Build history of the part. All positions in model axes, mm. A direction names the side the tool comes from. Round coordinates to 2 decimals unless told otherwise and drop trailing zeros. Write each loop counter-clockwise with the first axis right and the second up, starting at its lowest first coordinate (ties: lowest second). Pieces come first, ordered by that corner, then holes. Notation, with made-up numbers: (41.25, 2) - (81.25, 2) arc R24 cw to (81.25, 14) - close; hole circle Ø2 at (-27, -21). An arc over 180 degrees is marked (long way). Write each question's results on one line, items separated by ' | '.
from build123d import *

# Parameters (mm, degrees)
ESQUISSE1_W             = 55
ESQUISSE1_H             = 55
ESQUISSE1_W_2           = 45
ESQUISSE1_H_2           = 45
BOSS_EXTRU_1_DEPTH      = 60
ESQUISSE2_R             = 2
ESQUISSE2_W             = 20.2
ESQUISSE2_H             = 40.3
ENL_V_MAT_EXTRU_1_DEPTH = 10
ESQUISSE5_R             = 10
ESQUISSE5_R_2           = 1.5
ENL_V_MAT_EXTRU_2_DEPTH = 10
ENL_V_MAT_EXTRU_3_DEPTH = 89.413584698


with BuildPart() as part:
    # Esquisse1 → Boss.-Extru.1 (new body)
    with BuildSketch(Plane.XY):
        with Locations((-19.082718041, 7.024802088)):
            Rectangle(ESQUISSE1_W, ESQUISSE1_H)
        with Locations((-19.082718041, 7.024802088)):
            Rectangle(ESQUISSE1_W_2, ESQUISSE1_H_2, mode=Mode.SUBTRACT)
    extrude(amount=BOSS_EXTRU_1_DEPTH)

    # Esquisse2 → Enlèv. mat.-Extru.1 (cut)
    with BuildSketch(Plane(origin=(0, 34.524802088, 0), x_dir=(1, 0, 0), z_dir=(0, 1, 0))):
        with Locations(Location((-24.082718041, -3.25, 0), (0, 0, 270))):
            Circle(ESQUISSE2_R)
        with Locations(Location((-14.082718041, -3.25, 0), (0, 0, 270))):
            Circle(ESQUISSE2_R)
        with Locations(Location((-24.082718041, -51.25, 0), (0, 0, 270))):
            Circle(ESQUISSE2_R)
        with Locations(Location((-14.082718041, -51.25, 0), (0, 0, 270))):
            Circle(ESQUISSE2_R)
        with Locations((-19.082718041, -27.25)):
            Rectangle(ESQUISSE2_W, ESQUISSE2_H)
    extrude(amount=-ENL_V_MAT_EXTRU_1_DEPTH, mode=Mode.SUBTRACT)

    # Esquisse5 → Enlèv. mat.-Extru.2 (cut)
    with BuildSketch(Plane.XZ.offset(20.475197912)):
        with Locations(Location((-19.082718041, 17.1, 0), (0, 0, 270))):
            Circle(ESQUISSE5_R)
        with Locations(Location((-31.197044543, 5.605084019, 0), (0, 0, 270))):
            Circle(ESQUISSE5_R_2)
        with Locations(Location((-6.968391539, 5.605084019, 0), (0, 0, 270))):
            Circle(ESQUISSE5_R_2)
        with Locations(Location((-31.197044543, 28.594915981, 0), (0, 0, 270))):
            Circle(ESQUISSE5_R_2)
        with Locations(Location((-6.968391539, 28.594915981, 0), (0, 0, 270))):
            Circle(ESQUISSE5_R_2)
    extrude(amount=-ENL_V_MAT_EXTRU_2_DEPTH, mode=Mode.SUBTRACT)

    # Esquisse8 → Enlèv. mat.-Extru.3 (cut, through all)
    with BuildSketch(Plane(origin=(8.417281959, 0, 0), x_dir=(0, 0, -1), z_dir=(1, 0, 0))):
        Polygon((-50, 27.024802088), (-12.828427125, 27.024802088), (-50, -9.859909005), align=None)
        Polygon((-47.383863207, -12.898988168), (-10, -12.898988168), (-10, 24.196374963), align=None)
    extrude(amount=-ENL_V_MAT_EXTRU_3_DEPTH, mode=Mode.SUBTRACT)


solid = part.part
(1) Drill centre lines: probe 1 along X at (y, z) = (32.3, 3.25); probe 2 along Y at (x, z) = (3, 29); probe 3 along Z at (x, y) = (5, -9.5). Where is each one in solid material? Low to high. Write a range as [from, to].
Worked answers:
probe 1: x = [-46.58, -26.08], [-22.08, -16.08], [-12.08, 8.42] | probe 2: y = [-20.48, -15.48], [29.52, 34.52] | probe 3: z = [0, 10], [43.96, 49.64], [50, 60]
(2) Tool access for faces 1 (the flat face through (-29.183, 32, 28)), 2 (the cylindrical face through (-7.54, -18.01, 27.21)), 3 (the flat face through (-19, -20.475, 30)), 4 (the flat face through (3.417, 7, 30)), 5 (the flat face through (5.95, 5.91, 28.43)): list every direction of +Z, -Z, +X, -X, +Y, -Y with a clear straight run to the whole face (end or side of a thin tool).
Worked answers:
face 1: +Y | face 2: -Y | face 3: +Z, -Z, +X, -X, -Y | face 4: +Z, -Z | face 5: +X, -X
(3) Slice it at B-B, the plane z = 3.25. Write the cut outline in (x, y).
Worked answers:
outline: (-46.58, -20.48) - (8.42, -20.48) - (8.42, 34.52) - (-12.08, 34.52) - (-12.08, 29.52) - (3.42, 29.52) - (3.42, -15.48) - (-41.58, -15.48) - (-41.58, 29.52) - (-26.08, 29.52) - (-26.08, 34.52) - (-46.58, 34.52) - close; (-22.08, 29.52) - (-16.08, 29.52) - (-16.08, 34.52) - (-22.08, 34.52) - close
(4) Slice it at A-A, the plane x = 0. Write the cut outline in (y, z).
Worked answers:
outline: (-20.48, 0) - (-15.48, 0) - (-15.48, 60) - (-20.48, 60) - close; (29.52, 0) - (34.52, 0) - (34.52, 60) - (29.52, 60) - close
(5) Two-plate mould, pull along X, no slides. Class faces 6 (the flat face through (8.417, 7, 30)), 7 (the cylindrical face through (-22.1, 32.1, 51)), 8 (the flat face through (-44, 7, 60)): released by +X, released by -X, zero draft, split by the parting line, or undercut.
Worked answers:
face 6: released by +X | face 7: undercut | face 8: zero draft
(6) Slice it at C-C, the plane y = 21. Write the cut outline in (x, z), and give its area (3 significant figures).
Worked answers:
outline: (-46.58, 0) - (-41.58, 0) - (-41.58, 10) - (-46.58, 10) - close; (-46.58, 13.22) - (-41.58, 13.22) - (-41.58, 18.9) - (-46.58, 18.9) - close; (-46.58, 50) - (-41.58, 50) - (-41.58, 60) - (-46.58, 60) - close; (3.42, 0) - (8.42, 0) - (8.42, 10) - (3.42, 10) - close; (3.42, 13.22) - (8.42, 13.22) - (8.42, 18.9) - (3.42, 18.9) - close; (3.42, 50) - (8.42, 50) - (8.42, 60) - (3.42, 60) - close | area: 257 mm2
(7) Flat gauge pins, fed straight in: pin 1 Ø12 at (y, z) = (5.5, 28.5) entering from +X; pin 2 Ø2 at (x, z) = (-21, 38.5) entering from +Y; pin 3 Ø2.5 at (x, z) = (-31.2, 5.61) entering from -Y; pin 4 Ø16 at (x, z) = (-19.08, 17.1) entering from +Y. Where does each tip first touch, or does it go through?
Worked answers:
pin 1: stops at x = 8.42 | pin 2: stops at y = -15.48 | pin 3: stops at y = 29.52 | pin 4: passes through
(8) Slice it at D-D, the plane z = 44. Write the cut outline in (x, y), and give its area (3 significant figures).
Worked answers:
outline: (-46.58, -20.48) - (8.42, -20.48) - (8.42, -12.9) - (3.42, -12.9) - (3.42, -15.48) - (-41.58, -15.48) - (-41.58, -12.9) - (-46.58, -12.9) - close; (-46.58, -9.54) - (-41.58, -9.54) - (-41.58, -3.91) - (-46.58, -3.91) - close; (-46.58, 27.02) - (-41.58, 27.02) - (-41.58, 29.52) - (-29.18, 29.52) - (-29.18, 34.52) - (-46.58, 34.52) - close; (-8.98, 29.52) - (3.42, 29.52) - (3.42, 27.02) - (8.42, 27.02) - (8.42, 34.52) - (-8.98, 34.52) - close; (3.42, -9.54) - (8.42, -9.54) - (8.42, -3.91) - (3.42, -3.91) - close | area: 556 mm2
